Solid Edge part; units mm, degrees
sketch "Sketch1" plane through (0, 0, 0) normal (0, 0, 1) x (1, 0, 0)
  line L0 (4, 0) -> (4, 12)
  line L1 (0, 12) -> (4, 12)
  line L2 (0, 0) -> (0, 12)
  line L3 (0, 0) -> (0, -4.4)
  line L4 (0, -4.4) -> (7, -4.4)
  line L5 (7, -4.4) -> (7, 0)
  line L6 (7, 0) -> (4, 0)
revolve "RevolvedProtrusion1" add sketch "Sketch1" angle 360 about axis through (0, 0, 0) along (0, 1, 0)
sketch "Sketch2" plane through (0, 0, 0) normal (1, 0, 0) x (0, 1, 0)
  line L0 (-4.4, 3.3615) -> (-1.8, 3.3615)
  line L1 (0.1408, 0) -> (-1.8, 3.3615)
  line L2 (-4.4, 0) -> (0.1408, 0)
  line L3 (-4.4, 0) -> (-4.4, 3.3615)
revolve "RevolvedCutout1" cut sketch "Sketch2" angle 360 about axis through (0, -4.5, 0) along (0, 1, 0)
sketch "Sketch3" plane through (0, -4.4, 0) normal (0, -1, 0) x (0, 0, 1)
  circle A0 centre (0, 0) radius 3.3615
  line L0 (-2.5, -1.4434) -> (0, -2.8868)
  line L1 (0, -2.8868) -> (2.5, -1.4434)
  line L2 (2.5, -1.4434) -> (2.5, 1.4434)
  line L3 (2.5, 1.4434) -> (0, 2.8868)
  line L4 (0, 2.8868) -> (-2.5, 1.4434)
  line L5 (-2.5, 1.4434) -> (-2.5, -1.4434)
extrude "Protrusion1" add sketch "Sketch3" against normal up to next
sketch "Sketch4" plane through (0, 0, 0) normal (0, 0, 1) x (1, 0, 0)
  line L0 (-2.8868, -4.4) -> (0, -4.4)
  line L1 (0, -4.4) -> (0, -3.6265)
  line L2 (0, -3.6265) -> (-2.8868, -4.4)
revolve "RevolvedCutout2" cut sketch "Sketch4" angle 360 about axis through (0, -4.5, 0) along (0, 1, 0)
fillet "Round1" radius 0.4 1 edges at (0, 0, -4)
chamfer "倒斜角_2" distance 0.5333 angle 45 1 edges at (0, 12, -4)
cosmetic_thread "螺纹_3" thread depth 9.5
sketch "Sketch5" plane through (0, 0, 0) normal (0, 0, 1) x (1, 0, 0)
  arc A0 (-3.8153, -4.4) -> (-7, 0) centre (-2.3681, 0) cw
revolve "RevolvedCutout3" cut sketch "Sketch5" angle 360 about axis through (0, 0, 0) along (0, -1, 0) material side at (-6.1609, -2.7452, 0)
Verification items for the finished model (mm, model axes). A direction names the side the tool comes from. Give positions to 0.01 mm unless a question says otherwise; leave off trailing zeros. Loops run counter-clockwise (first coordinate to the right, second up) from the corner with the lowest first, then second, coordinate; pieces in that order, holes last. Notation, with made-up numbers: (-29, 77.25) - (-13, 77.25) arc R6 ccw to (-13, 81.25) - close; hole circle Ø2 at (-1, 25). An arc over 180 degrees is marked (long way). Write item = value, one per line. Start each with the question number.
Q1. Cross-section at A-A, the plane y = 10. Enter the section's corners in (x, z), and give its area (3 significant figures).
Q2. Tool access check on faces 1 (the face through (2.175, -2.873, 1.233)), 2 (the face through (0, 0, 5)), 3 (the face through (-3, -4.4, 1)). Record the directions out of +Z, -Z, +X, -X, +Y, -Y that give a thin tool (end or side, any length) a straight path to the whole face; none if there is none.
Q3. Thickness scan on line 1 (Z direction, x = -2, y = 3.25); line 2 (Y direction, x = -0.5, z = -5.5); line 3 (Y direction, x = -3.25, z = -5.75). Record the ranges inside material, lowest first.
Q4. Depth check by flat-ended pin: P1, Ø2, axis at x = 4.5, z = -4.5, coming from the +Y side; P2, Ø3, axis at x = -0.5, y = -3, coming from the +Z side; P3, Ø3, axis at x = 0.5, y = -3.5, coming from the -Z side. Enter the tip coordinate at first touch or a pass-through.
Q5. Mould release check, pull along Z, two halves, no side actions. Record for faces 4 (the face through (-0.867, 6.011, 3.905)), 5 (the face through (0, 12, 0)), 6 (the face through (-0.058, -4.337, -2.652)): released by +Z, released by -Z, zero draft, split by the parting line, or undercut.
Answer key:
q1.outline = circle Ø8 at (0, 0)
q1.area = 50.3 mm^2
q2.face_1 = -Y
q2.face_2 = +Y
q2.face_3 = +Z, -Z, +X, -X, -Y
q3.line_1 = -3.46 to 3.46
q3.line_2 = -3.39 to 0
q3.line_3 = -1.87 to 0
q4.P1 = 0
q4.P2 = 6.74
q4.P3 = -6.53
q5.face_4 = split by the parting line
q5.face_5 = zero draft
q5.face_6 = undercut
